```python
from build123d import *

# Parameters (mm, degrees)
SKETCH1_R           = 1.905
BOSS_EXTRUDE1_DEPTH = 4.318


with BuildPart() as part:
    # Sketch1 → Boss-Extrude1 (new body)
    with BuildSketch(Plane(origin=(0, 0, 0), x_dir=(0, 0, -1), z_dir=(1, 0, 0))):
        with BuildLine():
            Line((16, 0), (74.195959493, 0))
            ThreePointArc((74.195959493, 0), (77.731493399, 1.464466094), (79.195959493, 5))
            Line((79.195959493, 5), (79.195959493, 65))
            Line((79.195959493, 65), (16, 65))
            ThreePointArc((16, 65), (4.686291501, 60.313708499), (0, 49))
            Line((0, 49), (0, 16))
            ThreePointArc((0, 16), (4.686291501, 4.686291501), (16, 0))
        make_face()
        with Locations((63.195959493, 57)):
            Circle(SKETCH1_R, mode=Mode.SUBTRACT)
        with Locations((63.195959493, 41)):
            Circle(SKETCH1_R, mode=Mode.SUBTRACT)
        with Locations((63.195959493, 25)):
            Circle(SKETCH1_R, mode=Mode.SUBTRACT)
    extrude(amount=-BOSS_EXTRUDE1_DEPTH)


solid = part.part
```
Check sheet for the modelled part. Datum: model origin and axes. Units: mm. Round coordinates to 2 decimals unless told otherwise and drop trailing zeros. Order: outer loops, then holes, each group sorted by start corner. A loop starts at its lowest first (then second) coordinate and runs counter-clockwise, first axis right, second up.
1) Mould release check, pull along Y, two halves, no side actions. Record for faces 1 (the cylindrical face through (-2.129, 60.437, -4.811)), 2 (the flat face through (-4.318, 33, -39)), 3 (the cylindrical face through (-2.129, 24.27, -64.956)): +Y half, -Y half, draft (parallel to the pull), parting line (faces both ways), or undercut.
2) Section check A-A (x = -2.5). Record the boundary of the cut face in (y, z) (3 decimals), and give its area (3 significant figures).
3) Section check B-B (y = 25). Record the boundary of the cut face in (x, z).
4) Go/stop test with flat-tipped pins: pin 1 Ø3 at (y, z) = (57, -63.2) entering from +X; pin 2 Ø5 at (y, z) = (41, -63.2) entering from -X. Record where each tip stops, or that it passes through.
5) Section check C-C (y = 57). Record the boundary of the cut face in (x, z), and give its area (3 significant figures).
6) Section check D-D (y = 9.5). Record the boundary of the cut face in (x, z).
7) Scan lines: line 1 (Y direction, x = -3.35, z = -64.5); line 2 (Z direction, x = -1.05, y = 26.5); line 3 (Z direction, x = -0.8, y = 4). Record each from-to range of solid material in increasing order.
Result:
1. face 1: +Y half
1. face 2: draft
1. face 3: undercut
2. outline: (0, -74.196) arc R5 ccw to (5, -79.196) - (65, -79.196) - (65, -16) arc R16 ccw to (49, 0) - (16, 0) arc R16 ccw to (0, -16) - close; hole circle Ø3.81 at (25, -63.196); hole circle Ø3.81 at (41, -63.196); hole circle Ø3.81 at (57, -63.196)
2. area: 5,000 mm2
3. outline: (-4.32, -79.2) - (0, -79.2) - (0, -65.1) - (-4.32, -65.1) - close; (-4.32, -61.29) - (0, -61.29) - (0, 0) - (-4.32, 0) - close
4. pin 1: passes through
4. pin 2: stops at x = -4.32
5. outline: (-4.32, -79.2) - (0, -79.2) - (0, -65.1) - (-4.32, -65.1) - close; (-4.32, -61.29) - (0, -61.29) - (0, -2.14) - (-4.32, -2.14) - close
5. area: 316 mm2
6. outline: (-4.32, -79.2) - (0, -79.2) - (0, -1.38) - (-4.32, -1.38) - close
7. line 1: y = 0 to 23.61, 26.39 to 39.61, 42.39 to 55.61, 58.39 to 65
7. line 2: z = -79.2 to -64.37, -62.02 to 0
7. line 3: z = -79.09 to -5.42
